from build123d import *

# Parameters (mm, degrees)
SKETCH1_W           = 6.35
SKETCH1_H           = 66.04
BOSS_EXTRUDE1_DEPTH = 6.35


with BuildPart() as part:
    # Sketch1 → Boss-Extrude1 (new body)
    with BuildSketch(Plane(origin=(0, 0, 0), x_dir=(0, 0, -1), z_dir=(1, 0, 0))):
        Polygon((-237.109, 0), (237.109, 0), (138.588815033, 76.2), (-237.109, 76.2), align=None)
        with Locations((-208.534, 38.1)):
            Rectangle(SKETCH1_W, SKETCH1_H, mode=Mode.SUBTRACT)
        with Locations((-221.234, 38.1)):
            Rectangle(SKETCH1_W, SKETCH1_H, mode=Mode.SUBTRACT)
        with Locations((-195.834, 38.1)):
            Rectangle(SKETCH1_W, SKETCH1_H, mode=Mode.SUBTRACT)
        with Locations((-183.134, 38.1)):
            Rectangle(SKETCH1_W, SKETCH1_H, mode=Mode.SUBTRACT)
        with Locations((-170.434, 38.1)):
            Rectangle(SKETCH1_W, SKETCH1_H, mode=Mode.SUBTRACT)
        with Locations((-157.734, 38.1)):
            Rectangle(SKETCH1_W, SKETCH1_H, mode=Mode.SUBTRACT)
        with Locations((-145.034, 38.1)):
            Rectangle(SKETCH1_W, SKETCH1_H, mode=Mode.SUBTRACT)
        with Locations((-132.334, 38.1)):
            Rectangle(SKETCH1_W, SKETCH1_H, mode=Mode.SUBTRACT)
        with Locations((-119.634, 38.1)):
            Rectangle(SKETCH1_W, SKETCH1_H, mode=Mode.SUBTRACT)
        with Locations((-106.934, 38.1)):
            Rectangle(SKETCH1_W, SKETCH1_H, mode=Mode.SUBTRACT)
        with Locations((-94.234, 38.1)):
            Rectangle(SKETCH1_W, SKETCH1_H, mode=Mode.SUBTRACT)
        with Locations((-81.534, 38.1)):
            Rectangle(SKETCH1_W, SKETCH1_H, mode=Mode.SUBTRACT)
        with Locations((-68.834, 38.1)):
            Rectangle(SKETCH1_W, SKETCH1_H, mode=Mode.SUBTRACT)
        with Locations((-56.134, 38.1)):
            Rectangle(SKETCH1_W, SKETCH1_H, mode=Mode.SUBTRACT)
        with Locations((-43.434, 38.1)):
            Rectangle(SKETCH1_W, SKETCH1_H, mode=Mode.SUBTRACT)
        with Locations((-30.734, 38.1)):
            Rectangle(SKETCH1_W, SKETCH1_H, mode=Mode.SUBTRACT)
        with Locations((-18.034, 38.1)):
            Rectangle(SKETCH1_W, SKETCH1_H, mode=Mode.SUBTRACT)
        with Locations((-5.334, 38.1)):
            Rectangle(SKETCH1_W, SKETCH1_H, mode=Mode.SUBTRACT)
        with Locations((7.366, 38.1)):
            Rectangle(SKETCH1_W, SKETCH1_H, mode=Mode.SUBTRACT)
        with Locations((20.066, 38.1)):
            Rectangle(SKETCH1_W, SKETCH1_H, mode=Mode.SUBTRACT)
        with Locations((32.766, 38.1)):
            Rectangle(SKETCH1_W, SKETCH1_H, mode=Mode.SUBTRACT)
        with Locations((45.466, 38.1)):
            Rectangle(SKETCH1_W, SKETCH1_H, mode=Mode.SUBTRACT)
        with Locations((58.166, 38.1)):
            Rectangle(SKETCH1_W, SKETCH1_H, mode=Mode.SUBTRACT)
        with Locations((70.866, 38.1)):
            Rectangle(SKETCH1_W, SKETCH1_H, mode=Mode.SUBTRACT)
        with Locations((83.566, 38.1)):
            Rectangle(SKETCH1_W, SKETCH1_H, mode=Mode.SUBTRACT)
        with Locations((96.266, 38.1)):
            Rectangle(SKETCH1_W, SKETCH1_H, mode=Mode.SUBTRACT)
        with Locations((108.966, 38.1)):
            Rectangle(SKETCH1_W, SKETCH1_H, mode=Mode.SUBTRACT)
        with Locations((121.666, 38.1)):
            Rectangle(SKETCH1_W, SKETCH1_H, mode=Mode.SUBTRACT)
        with Locations((134.366, 38.1)):
            Rectangle(SKETCH1_W, SKETCH1_H, mode=Mode.SUBTRACT)
    extrude(amount=-BOSS_EXTRUDE1_DEPTH)


solid = part.part
Geometry check sheet. Reference: the model listing, model coordinates, mm. Round coordinates to 2 decimals unless told otherwise and drop trailing zeros. Order: outer loops, then holes, each group sorted by start corner. A loop starts at its lowest first (then second) coordinate and runs counter-clockwise, first axis right, second up. Notation, with made-up numbers: (-1, -28) - (41, -28) arc R15 cw to (41, -16) - close; hole circle Ø5 at (19, 34). An arc over 180 degrees is marked (long way). One line per question, with ' | ' between items. Start each with the question number.
(1) Depth check by flat-ended pin: pin 1 Ø1.9 at (x, y) = (-3, 38) entering from -Z; pin 2 Ø1.9 at (x, y) = (-2, 24.5) entering from -Z. Enter the tip coordinate at first touch or a pass-through.
(2) Sectioned sample at C-C on z = -180. Record the cut outline in (x, y), and give its area (3 significant figures).
(3) Thickness scan on L1, parallel to Y at x = -5.25, z = 156; L2, parallel to Y at x = -3.5, z = -187; L3, parallel to Y at x = -1.75, z = -169. Record the ranges inside material, lowest first. Write a range as [from, to].
(4) Sectioned sample at A-A on x = -3.5. Count the separate pieces of the cut face and the enclosed holes in it, and give its area (3 significant figures).
Conclusion:
1) pin 1: stops at z = -189.21 | pin 2: stops at z = -206.66
2) outline: (-6.35, 0) - (0, 0) - (0, 44.17) - (-6.35, 44.17) - close | area: 280 mm2
3) L1: y = [0, 5.08], [71.12, 76.2] | L2: y = [0, 38.76] | L3: y = [0, 52.68]
4) separate pieces: 1 | enclosed holes: 29 | area: 20,200 mm2
